The model under review builds one solid part; all positions refer to its coordinate system, in mm. A direction names the side the tool comes from. Coordinates: 2 decimals unless noted, no trailing zeros. Loops run counter-clockwise (first coordinate to the right, second up) from the corner with the lowest first, then second, coordinate; pieces in that order, holes last. Notation, with made-up numbers: M 6,25 L 11,25 A28 cw 11,64 Z; hole C 67,-10.5 d4. An arc over 180 degrees is marked long. One line per item, written item: value.
```python
from build123d import *

# Parameters (mm, degrees)
F1_DEPTH = 0.8
F2_W     = 76.2
F2_H     = 213.36
F2_W_2   = 74.6
F2_H_2   = 20.776
F2_H_3   = 20.376
F3_DEPTH = 44
F4_R     = 0.4
F5_DEPTH = 0.8


with BuildPart() as f1:
    # F0 (on Top) → F1 (new body)
    with BuildSketch(Plane.XY):
        with BuildLine():
            Line((0, 12.5), (0, 0))
            Line((0, 0), (12.5, 0))
            ThreePointArc((12.5, 0), (8.8388347648, 8.8388347648), (0, 12.5))
        make_face()
        with BuildLine():
            ThreePointArc((0, 12.5), (8.8388347648, 8.8388347648), (12.5, 0))
            Line((12.5, 0), (63.7, 0))
            ThreePointArc((63.7, 0), (67.3611652352, 8.8388347648), (76.2, 12.5))
            Line((76.2, 12.5), (76.2, 200.86))
            ThreePointArc((76.2, 200.86), (67.3611652352, 204.5211652352), (63.7, 213.36))
            Line((63.7, 213.36), (12.5, 213.36))
            ThreePointArc((12.5, 213.36), (8.8388347648, 204.5211652352), (0, 200.86))
            Line((0, 200.86), (0, 12.5))
        make_face()
        with BuildLine():
            ThreePointArc((76.2, 12.5), (67.3611652352, 8.8388347648), (63.7, 0))
            Line((63.7, 0), (76.2, 0))
            Line((76.2, 0), (76.2, 12.5))
        make_face()
        with BuildLine():
            ThreePointArc((63.7, 213.36), (67.3611652352, 204.5211652352), (76.2, 200.86))
            Line((76.2, 200.86), (76.2, 213.36))
            Line((76.2, 213.36), (63.7, 213.36))
        make_face()
        with BuildLine():
            Line((0, 213.36), (0, 200.86))
            ThreePointArc((0, 200.86), (8.8388347648, 204.5211652352), (12.5, 213.36))
            Line((12.5, 213.36), (0, 213.36))
        make_face()
    extrude(amount=F1_DEPTH)

    # F2 (on face) → F3 (join)
    with BuildSketch(Plane.XY.offset(0.8)):
        with Locations((38.1, 106.68)):
            Rectangle(F2_W, F2_H)
        with Locations((38.1, 11.188)):
            Rectangle(F2_W_2, F2_H_2, mode=Mode.SUBTRACT)
        with Locations((38.1, 32.564)):
            Rectangle(F2_W_2, F2_H_3, mode=Mode.SUBTRACT)
        with Locations((38.1, 53.74)):
            Rectangle(F2_W_2, F2_H_3, mode=Mode.SUBTRACT)
        with Locations((38.1, 74.916)):
            Rectangle(F2_W_2, F2_H_3, mode=Mode.SUBTRACT)
        with Locations((38.1, 96.092)):
            Rectangle(F2_W_2, F2_H_3, mode=Mode.SUBTRACT)
        with Locations((38.1, 117.268)):
            Rectangle(F2_W_2, F2_H_3, mode=Mode.SUBTRACT)
        with Locations((38.1, 138.444)):
            Rectangle(F2_W_2, F2_H_3, mode=Mode.SUBTRACT)
        with Locations((38.1, 159.62)):
            Rectangle(F2_W_2, F2_H_3, mode=Mode.SUBTRACT)
        with Locations((38.1, 180.796)):
            Rectangle(F2_W_2, F2_H_3, mode=Mode.SUBTRACT)
        with Locations((38.1, 202.172)):
            Rectangle(F2_W_2, F2_H_2, mode=Mode.SUBTRACT)
    extrude(amount=F3_DEPTH)

    # F4
    f4_edges = [f1.edges().sort_by_distance(p)[0] for p in [
        (75.4, 0.8, 22.8),
        (76.2, 0, 22.4),
        (0.8, 0.8, 22.8),
        (0, 0, 22.4),
        (0, 213.36, 22.4),
        (0.8, 212.56, 22.8),
        (76.2, 213.36, 22.4),
        (75.4, 212.56, 22.8),
    ]]
    fillet(f4_edges, radius=F4_R)

    # F0 (on Top) → F5 (join, through all)
    with BuildSketch(Plane.XY):
        with BuildLine():
            Line((76.2, 0), (63.7, 0))
            ThreePointArc((63.7, 0), (76.2, -12.5), (88.7, 0))
            ThreePointArc((88.7, 0), (85.0388347648, 8.8388347648), (76.2, 12.5))
            Line((76.2, 12.5), (76.2, 0))
        make_face()
        with BuildLine():
            Line((12.5, 0), (0, 0))
            Line((0, 0), (0, 12.5))
            ThreePointArc((0, 12.5), (-8.8388347648, -8.8388347648), (12.5, 0))
        make_face()
        with BuildLine():
            ThreePointArc((12.5, 213.36), (-8.8388347648, 222.1988347648), (0, 200.86))
            Line((0, 200.86), (0, 213.36))
            Line((0, 213.36), (12.5, 213.36))
        make_face()
        with BuildLine():
            Line((76.2, 213.36), (76.2, 200.86))
            ThreePointArc((76.2, 200.86), (85.0388347648, 204.5211652352), (88.7, 213.36))
            ThreePointArc((88.7, 213.36), (76.2, 225.86), (63.7, 213.36))
            Line((63.7, 213.36), (76.2, 213.36))
        make_face()
        with BuildLine():
            ThreePointArc((76.2, 12.5), (67.3611652352, 8.8388347648), (63.7, 0))
            Line((63.7, 0), (76.2, 0))
            Line((76.2, 0), (76.2, 12.5))
        make_face()
        with BuildLine():
            Line((0, 12.5), (0, 0))
            Line((0, 0), (12.5, 0))
            ThreePointArc((12.5, 0), (8.8388347648, 8.8388347648), (0, 12.5))
        make_face()
        with BuildLine():
            Line((0, 213.36), (0, 200.86))
            ThreePointArc((0, 200.86), (8.8388347648, 204.5211652352), (12.5, 213.36))
            Line((12.5, 213.36), (0, 213.36))
        make_face()
        with BuildLine():
            ThreePointArc((63.7, 213.36), (67.3611652352, 204.5211652352), (76.2, 200.86))
            Line((76.2, 200.86), (76.2, 213.36))
            Line((76.2, 213.36), (63.7, 213.36))
        make_face()
    extrude(amount=F5_DEPTH)


solid = f1.part
```
(1) Insertion check: pin 1 Ø6 at (x, y) = (31, 15.5) entering from +Z; pin 2 Ø16.5 at (y, z) = (181, 24.5) entering from +X; pin 3 Ø6 at (x, z) = (2.5, 21.5) entering from +Y. Each pin has a flat end and moves straight along its axis. Give the tip position at first contact, or say it passes through.
Checks:
pin 1: z = 0.8
pin 2: x = 76.2
pin 3: y = 213.36
(2) Add section B-B on z = 14.5. State how many separate pieces and enclosed holes the cut face has, then the cut area to 3 significant figures.
Checks:
separate pieces: 1
enclosed holes: 10
area: 998 mm^2
(3) Draft analysis for pull direction X (two halves, no side actions). For faces 1 (the face through (0.8, 202, 22)), 2 (the face through (-3, -3, 0.8)), state which applies: pulls with the +X half, pulls with the -X half, needs draft (parallel to the pull), parting line crosses it, or undercut.
Checks:
face 1: undercut
face 2: needs draft
(4) Tool access review of faces 3 (the face through (38, 170.608, 22)), 4 (the face through (-9.13, -8.54, 0.39)): name each direction out of +Z, -Z, +X, -X, +Y, -Y from which nothing blocks a thin tool from reaching the whole face with its end or side.
Checks:
face 3: +Z
face 4: +Z, -Z
(5) Add section A-A on y = 67. State the section outline as (x, z) points.
Checks:
outline: M 0,0 L 76.2,0 L 76.2,44.8 L 75.4,44.8 L 75.4,0.8 L 0.8,0.8 L 0.8,44.8 L 0,44.8 Z
(6) To check wall thickness, follow L1, parallel to X at y = 154, z = 10.5; L2, parallel to Z at x = 68, y = 96. State the ranges of each line that lie inside material, in increasing order. Write a range as [from, to].
Checks:
L1: [0, 0.8], [75.4, 76.2]
L2: [0, 0.8]
